Verification items for this drawing (mm, ordinates from the low corner). A direction names the side the tool comes from. Give positions to 0.01 mm unless a question says otherwise; leave off trailing zeros. Loops run counter-clockwise (first coordinate to the right, second up) from the corner with the lowest first, then second, coordinate; pieces in that order, holes last. Notation, with made-up numbers: (52, 22.5) -> (73, 22.5) arc R21 ccw to (73, 53.5) -> close; hole circle Ø5 at (-24, 30.5). An arc over 180 degrees is marked (long way). Write item = value, one per line.
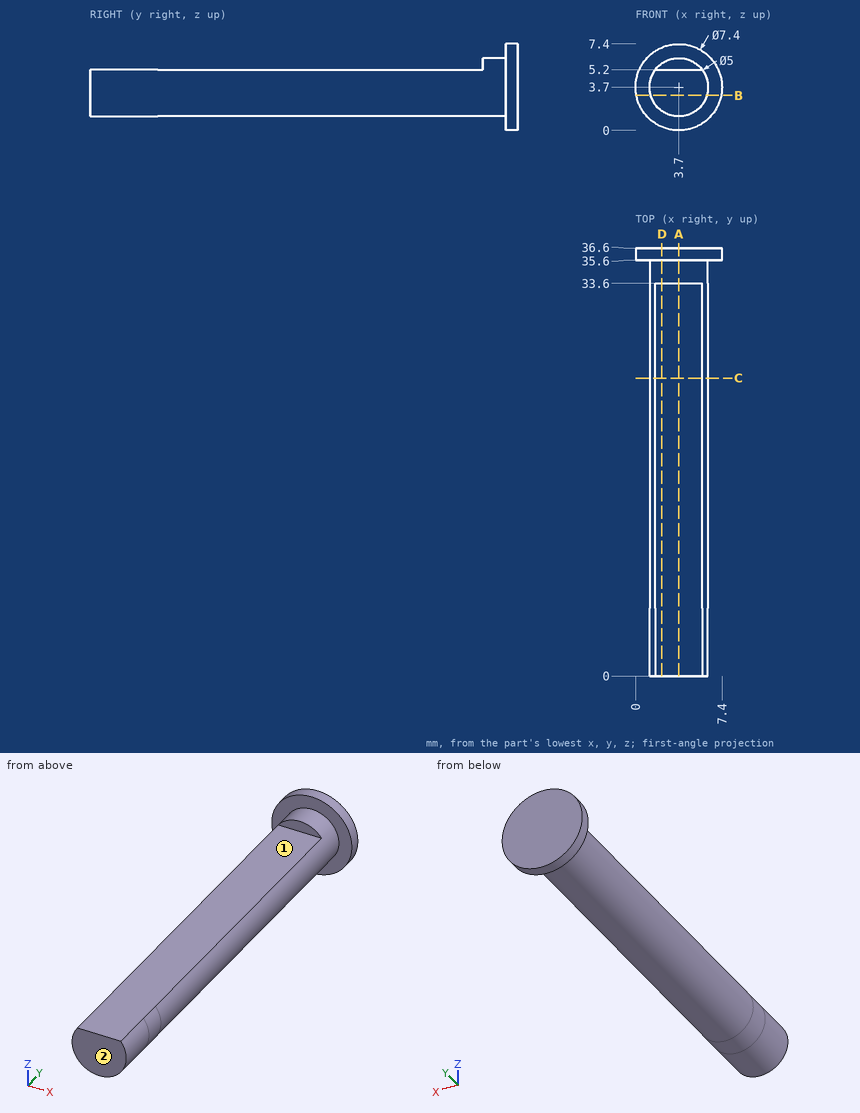
Item 1: Section check A-A, the plane x = 3.7. Record the cut outline in (y, z).
Answer:
outline = (0, 1.2) -> (35.6, 1.2) -> (35.6, 0) -> (36.6, 0) -> (36.6, 7.4) -> (35.6, 7.4) -> (35.6, 6.2) -> (33.6, 6.2) -> (33.6, 5.2) -> (0, 5.2) -> close
Item 2: Thickness scan on L1, parallel to Y at x = 3.25, z = 5.5; L2, parallel to Y at x = 2.5, z = 6.5; L3, parallel to X at y = 33.5, z = 3.75. Record the ranges inside material, lowest first. Write a range as [from, to].
Answer:
L1 = [33.6, 36.6]
L2 = [35.6, 36.6]
L3 = [1.2, 6.2]
Item 3: Section check B-B, the plane z = 3. Record the cut outline in (x, y).
Answer:
outline = (0.07, 35.6) -> (1.3, 35.6) -> (1.3, 0) -> (6.1, 0) -> (6.1, 35.6) -> (7.33, 35.6) -> (7.33, 36.6) -> (0.07, 36.6) -> close
Item 4: Gauge pin test, flat ends, axial feed: pin 1 (3 mm diameter, centred on x = 1, y = 4.5, fed in from -Z); pin 2 (1.5 mm diameter, centred on x = 3.5, y = 6, fed in from -Z); pin 3 (1.5 mm diameter, centred on x = 6.5, y = 12.5, fed in from +Z). Record the tip position at first contact, or that the pin passes through.
Answer:
pin_1 = 1.51
pin_2 = 1.2
pin_3 = 5.13
Item 5: Tool access check on the marked faces 1 and 2. Record the directions out of +Z, -Z, +X, -X, +Y, -Y that give a thin tool (end or side, any length) a straight path to the whole face; none if there is none.
Answer:
face_1 = +Z, +X, -X, -Y
face_2 = +Z, -Z, +X, -X, -Y
Item 6: Section check D-D, the plane x = 2.25. Record the cut outline in (y, z), plus the area to 3 significant figures.
Answer:
outline = (0, 1.66) -> (35.6, 1.66) -> (35.6, 0.3) -> (36.6, 0.3) -> (36.6, 7.1) -> (35.6, 7.1) -> (35.6, 5.74) -> (33.6, 5.74) -> (33.6, 5.2) -> (0, 5.2) -> close
area = 134 mm^2
Item 7: Section check C-C, the plane y = 25.5. Record the cut outline in (x, z).
Answer:
outline = (1.7, 5.2) arc R2.5 ccw (long way) to (5.7, 5.2) -> close
